Solid Edge part; units mm, degrees
sketch "Sketch1" plane through (0, 0, 0) normal (0, 0, 1) x (1, 0, 0)
  line L0 (-6, -1.3) -> (6, -1.3)
  line L1 (6, -1.3) -> (6, 1.3)
  line L2 (6, 1.3) -> (-6, 1.3)
  line L3 (-6, 1.3) -> (-6, -1.3)
  dimension "D1" = 6
extrude "Protrusion1" add sketch "Sketch1" along normal mid plane 2.6
sketch "Sketch2" plane through (6, 0, 0) normal (1, 0, 0) x (0, 1, 0)
  line L0 (-0.3, -0.3) -> (0.3, -0.3)
  line L1 (0.3, -0.3) -> (0.3, 0.3)
  line L2 (0.3, 0.3) -> (-0.3, 0.3)
  line L3 (-0.3, 0.3) -> (-0.3, -0.3)
  dimension "D1" = 0.3
  dimension "D2" = 0.3
extrude "Extrusionsausschnitt_1" cut sketch "Sketch2" against normal blind 5.5
chamfer "Fase_1" distance 0.5 angle 45 4 edges at (6, 0, 0.3) (6, 0.3, 0) (6, -0.3, 0) (6, 0, -0.3)
sketch "Sketch3" plane through (-6, 0, 0) normal (-1, 0, 0) x (0, -1, 0)
  circle A0 centre (0, 0) radius 0.75
extrude "Extrusionsausschnitt_2" cut sketch "Sketch3" against normal blind 5.5
sketch "Sketch4" plane through (0, 0, 1.3) normal (0, 0, 1) x (1, 0, 0)
  line L0 (0.2, -1.3) -> (-3.4, -1.3)
  line L1 (-3.4, -1.3) -> (-3.4, -0.7966)
  line L2 (-3.4, -0.7966) -> (0.2, -0.7966)
  line L3 (0.2, 0.8) -> (0.2, -0.7966)
  line L4 (-3.4, 0.8) -> (0.2, 0.8)
  line L5 (-3.4, 1.3) -> (-3.4, 0.8)
  line L6 (0.2, 1.3) -> (-3.4, 1.3)
  line L7 (2.4, 1.3) -> (0.2, 1.3)
  line L8 (2.4, -1.3) -> (2.4, 1.3)
  line L9 (0.2, -1.3) -> (2.4, -1.3)
  dimension "D1" = 2.4
  dimension "D2" = 3.4
  dimension "D3" = 3.4
  dimension "D4" = 0.2
extrude "Extrusionsausschnitt_3" cut sketch "Sketch4" against normal blind 0.1
sketch "Sketch5" plane through (-0.5, 0, 1.2) normal (0, 0, 1) x (1, 0, 0)
  line L0 (0.8, 0.8) -> (2.8, 0.8)
  line L1 (2.8, 0.8) -> (2.8, -0.8)
  line L2 (2.8, -0.8) -> (0.8, -0.8)
  line L3 (0.8, -0.8) -> (0.8, 0.8)
  dimension "D1" = 0.8
extrude "Extrusionsausschnitt_4" cut sketch "Sketch5" against normal blind 0.1
chamfer "Fase_2" distance 0.25 angle 45 1 edges at (-6, 0.75, 0)
Part model, mm, in its own coordinate system. A direction names the side the tool comes from. Give positions to 0.01 mm unless a question says otherwise; leave off trailing zeros. Write each loop counter-clockwise with the first axis right and the second up, starting at its lowest first coordinate (ties: lowest second). Pieces come first, ordered by that corner, then holes. Notation, with made-up numbers: (14, -7) -> (71, -7) arc R15 cw to (71, 5) -> close; hole circle Ø5 at (5, 59.25). An arc over 180 degrees is marked (long way). Put each result on its own line as item: value. Start each with the question number.
Item 1: Cut at A-A (x = 4.75). List the corners of the cut face in (y, z).
Item 2: Which spindle directions (+Z, -Z, +X, -X, +Y, -Y) get a long thin tool onto all of the face, cutting with end or side? Do faces 4 (the face through (-6, 1, -1)), 5 (the face through (-3.16, 0.75, 0.03)). Say none if no direction does.
Item 3: Pin check, flat tips, straight feed: pin 1 Ø0.5 at (y, z) = (0, 0) entering from +X; pin 2 Ø0.5 at (x, y) = (1.5, 0) entering from +Z. Stop position of each tip, or through.
Item 4: Cut at D-D (x = -3.75). List the corners of the cut face in (y, z).
Item 5: Cut at C-C (z = 0). List the corners of the cut face in (x, y).
Item 6: Wall check: L1, parallel to Z at x = -1.9, y = 0; L2, parallel to Z at x = 0.75, y = 0.15. Give the ranges that are in metal, low to high. Write a range as [from, to].
Item 7: Pull direction X, two halves, no side cores. Call faces 1 (the face through (-0.5, 0, 0)), 2 (the face through (1, 0, 1.1)), 3 (the face through (-4, 0, 1.3)): pulls with the +X half, pulls with the -X half, needs draft (parallel to the pull), parting line crosses it, or undercut.
Item 8: Cut at B-B (y = 0). List the corners of the cut face in (x, z), then the cut area to 3 significant figures.
Answer list:
1. outline: (-1.3, -1.3) -> (1.3, -1.3) -> (1.3, 1.3) -> (-1.3, 1.3) -> close; hole (-0.3, -0.3) -> (0.3, -0.3) -> (0.3, 0.3) -> (-0.3, 0.3) -> close
2. face 4: +Z, -Z, -X, +Y, -Y
2. face 5: -X
3. pin 1: stops at x = 0.5
3. pin 2: stops at z = 1.1
4. outline: (-1.3, -1.3) -> (1.3, -1.3) -> (1.3, 1.3) -> (-1.3, 1.3) -> close; hole circle Ø1.5 at (0, 0)
5. outline: (-6, -1.3) -> (6, -1.3) -> (6, -0.8) -> (5.5, -0.3) -> (0.5, -0.3) -> (0.5, 0.3) -> (5.5, 0.3) -> (6, 0.8) -> (6, 1.3) -> (-6, 1.3) -> (-6, 1) -> (-5.75, 0.75) -> (-0.5, 0.75) -> (-0.5, -0.75) -> (-5.75, -0.75) -> (-6, -1) -> close
6. L1: z = [-1.3, -0.75], [0.75, 1.3]
6. L2: z = [-1.3, -0.3], [0.3, 1.1]
7. face 1: pulls with the -X half
7. face 2: undercut
7. face 3: needs draft
8. outline: (-6, -1.3) -> (6, -1.3) -> (6, -0.8) -> (5.5, -0.3) -> (0.5, -0.3) -> (0.5, 0.3) -> (5.5, 0.3) -> (6, 0.8) -> (6, 1.3) -> (2.4, 1.3) -> (2.4, 1.2) -> (2.3, 1.2) -> (2.3, 1.1) -> (0.3, 1.1) -> (0.3, 1.2) -> (0.2, 1.2) -> (0.2, 1.3) -> (-6, 1.3) -> (-6, 1) -> (-5.75, 0.75) -> (-0.5, 0.75) -> (-0.5, -0.75) -> (-5.75, -0.75) -> (-6, -1) -> close
8. area: 18.9 mm2
